Work out the finished part from the listing and answer in its coordinate system (mm). Face numbers are marked on the shaded views. A direction names the side the tool comes from. Give positions to 0.01 mm unless a question says otherwise; leave off trailing zeros. Loops run counter-clockwise (first coordinate to the right, second up) from the corner with the lowest first, then second, coordinate; pieces in that order, holes last. Notation, with made-up numbers: M -14,-38 L 5,-38 A23 ccw 5,-6 Z; hole C 61,-30.5 d7. An arc over 180 degrees is marked long. Answer as a JSON object with one key per item and string values. Group by question number.
```python
from build123d import *

# Parameters (mm, degrees)
F0_R     = 5
F0_R_2   = 3.75
F0_R_3   = 2.5
F1_DEPTH = 20
F2_DEPTH = 12.5
F4_DEPTH = 5
F5_DEPTH = 20.001


with BuildPart() as f1:
    # F0 (on Top) → F1 (new body)
    with BuildSketch(Plane.XY):
        Polygon((0, 7.4358002841), (0, -22.5641997159), (50, -22.5641997159), (50, -12.5641997159), (5, 22.4358002841), (-20, 22.4358002841), (-20, 2.4358002841), (-15, 2.4358002841), (-15, 7.4358002841), align=None)
        with Locations((12.5, -12.5641997159)):
            Circle(F0_R, mode=Mode.SUBTRACT)
        with Locations((25.75, -12.5641997159)):
            Circle(F0_R_2, mode=Mode.SUBTRACT)
        with Locations((37.5, -12.5641997159)):
            Circle(F0_R_3, mode=Mode.SUBTRACT)
        with Locations((12.5, -12.5641997159)):
            Circle(F0_R)
        with Locations((25.75, -12.5641997159)):
            Circle(F0_R_2)
        with Locations((37.5, -12.5641997159)):
            Circle(F0_R_3)
    extrude(amount=-F1_DEPTH)

    # F0 (on Top) → F2 (cut, symmetric)
    with BuildSketch(Plane.XY):
        with Locations((12.5, -12.5641997159)):
            Circle(F0_R)
        with Locations((25.75, -12.5641997159)):
            Circle(F0_R_2)
        with Locations((37.5, -12.5641997159)):
            Circle(F0_R_3)
    extrude(amount=F2_DEPTH, both=True, mode=Mode.SUBTRACT)

    # F3 (on face) → F4 (cut)
    with BuildSketch(Plane(origin=(0, 0, -20), x_dir=(1, 0, 0), z_dir=(0, 0, -1))):
        Polygon((20.7619503973, 0), (23.1309751987, 0), (24.3154875993, 2.0516356601), (23.1309751987, 2.7355142135), (22.0358983849, 2.1032713203), (21.9762746603, 2), (21.8570272111, 2), (20.7619503973, 1.3677571068), align=None)
        Polygon((20.7619503973, -1.3677571068), (20.7619503973, 0), (18.7619503973, 0), (18.7619503973, -2.5224576451), (23.1309751987, -5.0449152903), (27.5, -2.5224576451), (27.5, 2.5224576451), (25.3154875993, 3.7836864677), (24.3154875993, 2.0516356601), (25.5, 1.3677571068), (25.5, -1.3677571068), (23.1309751987, -2.7355142135), align=None)
        Polygon((18.7619503973, 0), (20.7619503973, 0), (20.7619503973, 1.3677571068), (21.8570272111, 2), (18.7619503973, 2), align=None)
        Polygon((23.1309751987, 2.7355142135), (24.3154875993, 2.0516356601), (25.3154875993, 3.7836864677), (23.5834367918, 4.7836864677), (22.0358983849, 2.1032713203), align=None)
        Polygon((14.3965897144, 0), (18.7619503973, 0), (18.7619503973, 2), (15.5512902527, 2), (12.338798049, 7.5641997159), (15.5512902527, 13.1283994317), (21.9762746603, 13.1283994317), (25.1887668641, 7.5641997159), (23.5834367918, 4.7836864677), (25.3154875993, 3.7836864677), (27.4981679408, 7.5641997159), (23.1309751987, 15.1283994317), (14.3965897144, 15.1283994317), (10.0293969722, 7.5641997159), align=None)
        Polygon((18.7619503973, 2.5224576451), (18.7619503973, 2), (21.8570272111, 2), (22.0358983849, 2.1032713203), (23.5834367918, 4.7836864677), (23.1309751987, 5.0449152903), align=None)
        Polygon((22.3340887545, 4.9830829416), (22.3218557052, 10.162153838), (17.3924863607, 11.7509404388), (14.358201612, 7.5537936626), (17.4122798502, 3.3710276983), align=None)
        Polygon((35.4952501059, 15.1283994317), (27.4952501059, 15.1283994317), (31.4952501059, 8.2001962014), align=None)
        Polygon((12.7505299598, -6.9282032303), (8.7505299598, 0), (4.7505299598, -6.9282032303), align=None)
        Polygon((0, -9.4358002841), (-15, -9.4358002841), (-17, -9.4358002841), (-17, -4.4358002841), (-18, -4.4358002841), (-18, -20.4358002841), (-15, -20.4358002841), (0, -20.4358002841), align=None)
    extrude(amount=-F4_DEPTH, mode=Mode.SUBTRACT)

    # F3 (on face) → F5 (cut, through all)
    with BuildSketch(Plane(origin=(0, 0, -20), x_dir=(1, 0, 0), z_dir=(0, 0, -1))):
        Polygon((0, -9.4358002841), (-15, -9.4358002841), (-17, -9.4358002841), (-17, -4.4358002841), (-18, -4.4358002841), (-18, -20.4358002841), (-15, -20.4358002841), (0, -20.4358002841), align=None)
    extrude(amount=-F5_DEPTH, mode=Mode.SUBTRACT)


solid = f1.part
```
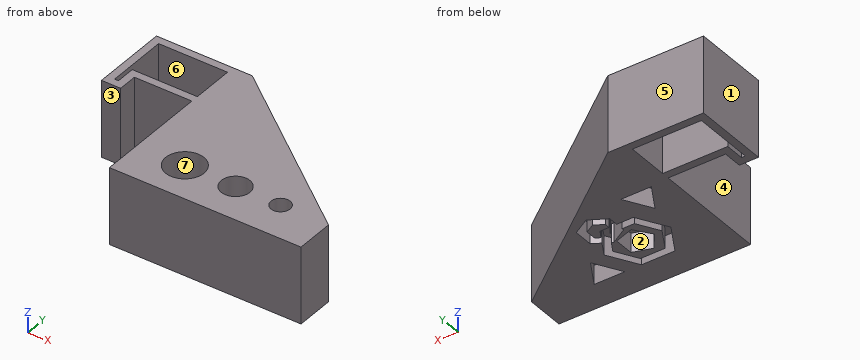
Item 1: Given pin 1 Ø1.5 at (x, z) = (16, -12) entering from +Y; pin 2 Ø1.1 at (y, z) = (0.5, -18.5) entering from -X; pin 3 Ø6 at (x, y) = (12.5, -12.56) entering from +Z, each flat-ended and moving along its own axis, determine where each tip first touches the part or whether it passes through.
Item 2: For a pull along Y with two mould halves and no side action, classify the marked faces 1, 2 and 3 as pulls with the +Y half, pulls with the -Y half, needs draft (parallel to the pull), parting line crosses it, or undercut.
Item 3: Find the intervals of material crossed by probe 1 along X at (y, z) = (1.5, -17.25); probe 2 along Y at (x, z) = (-6, -7); probe 3 along X at (y, z) = (3, -13.25), in increasing order. Write a range as [from, to].
Item 4: A cutting plane is placed at C-C (x = 33.5). Determine the outline of the cut face in (y, z), and give its area (3 significant figures).
Item 5: A tool of negligible diameter and unlimited length cuts with its end or side. For the marked faces 4, 5, 6 and 7, from which of +Z, -Z, +X, -X, +Y, -Y can it reach the whole face along a straight path? Write none if from no direction.
Item 6: A cutting plane is placed at A-A (z = -14.25). Determine the outline of the cut face in (x, y).
Item 7: A cutting plane is placed at B-B (z = -3). Determine the outline of the cut face in (x, y).
The answers:
{
 "1": {"pin 1": "stops at y = 14.46", "pin 2": "stops at x = 0", "pin 3": "stops at z = -12.5"},
 "2": {"face 1": "needs draft", "face 2": "undercut", "face 3": "pulls with the -Y half"},
 "3": {"probe 1": "x = [0, 7.88], [9.62, 18.76], [20.99, 25.27], [27.5, 31.92]", "probe 2": "y = [7.44, 9.44], [20.44, 22.44]", "probe 3": "x = [-20, -15], [0, 29.99]"},
 "4": {"outline": "M -22.56,-20 L -15.13,-20 L -15.13,-15 L -11.67,-15 L -11.67,-20 L 0.27,-20 L 0.27,0 L -22.56,0 Z", "area": "439 mm^2"},
 "5": {"face 4": "+Z, -Z, -Y", "face 5": "+Z, -Z, +X, -X, +Y", "face 6": "+Z, -Z", "face 7": "+Z"},
 "6": {"outline": "M -20,2.44 L -15,2.44 L -15,7.44 L 0,7.44 L 0,-22.56 L 50,-22.56 L 50,-12.56 L 5,22.44 L -20,22.44 Z; hole M -18,4.44 L -17,4.44 L -17,9.44 L 0,9.44 L 0,20.44 L -18,20.44 Z"},
 "7": {"outline": "M -20,2.44 L -15,2.44 L -15,7.44 L 0,7.44 L 0,-22.56 L 50,-22.56 L 50,-12.56 L 5,22.44 L -20,22.44 Z; hole M -18,4.44 L -17,4.44 L -17,9.44 L 0,9.44 L 0,20.44 L -18,20.44 Z; hole C 12.5,-12.56 d10; hole C 25.75,-12.56 d7.5; hole C 37.5,-12.56 d5"}
}
